```python
from build123d import *

# Parameters (mm, degrees)
SKETCH1_W           = 10
SKETCH1_H           = 10
BOSS_EXTRUDE1_DEPTH = 15
CUT_EXTRUDE1_DEPTH  = 0.3


with BuildPart() as part:
    # Sketch1 → Boss-Extrude1 (new body)
    with BuildSketch(Plane(origin=(0, 0, 0), x_dir=(1, 0, 0), z_dir=(0, 1, 0))):
        Rectangle(SKETCH1_W, SKETCH1_H)
        with BuildLine():
            Line((-1.658312395, 2.5), (1.658312395, 2.5))
            ThreePointArc((1.658312395, 2.5), (0, -3.043965134), (-1.658312395, 2.5))
        make_face(mode=Mode.SUBTRACT)
    extrude(amount=BOSS_EXTRUDE1_DEPTH)

    # Sketch2 → Cut-Extrude1 (cut)
    with BuildSketch(Plane.XY.offset(5)):
        with BuildLine():
            Line((-1.296362428, 9.754838654), (-0.6134698, 9.754838654))
            add(Edge.make_bspline(
                [(-0.6134698, 9.754838654), (-0.580041322, 9.754662904), (-0.515248611, 9.754322256), (-0.42102917, 9.749039125), (-0.332780359, 9.741835455), (-0.250476587, 9.730405362), (-0.174155884, 9.716613585), (-0.103588247, 9.699911769), (-0.038998075, 9.679885155), (0.038114662, 9.648038874), (0.126035323, 9.600715706), (0.221233715, 9.530787141), (0.302637955, 9.445254678), (0.372824272, 9.348772022), (0.428625391, 9.24263625), (0.468994689, 9.129377062), (0.494552564, 9.01045532), (0.497180998, 8.928812142), (0.498509367, 8.887550994)],
                knots=[0, 0, 0, 0, 0.00010027, 0.000194349, 0.000283026, 0.000365821, 0.000443519, 0.000515622, 0.000583254, 0.00064614, 0.000765662, 0.000881909, 0.000998927, 0.001118415, 0.001238844, 0.00135727, 0.001478274, 0.001601912, 0.001601912, 0.001601912, 0.001601912], degree=3))
            add(Edge.make_bspline(
                [(0.498509367, 8.887550994), (0.497416148, 8.848898438), (0.495267871, 8.772942521), (0.474725112, 8.661848412), (0.442564443, 8.556097193), (0.397859194, 8.456074808), (0.339757198, 8.364041195), (0.270898879, 8.279253929), (0.187822077, 8.205302872), (0.125578837, 8.163959969), (0.093962091, 8.142959648)],
                knots=[0, 0, 0, 0, 0.000115857, 0.00022767, 0.000337672, 0.000446877, 0.000555233, 0.000663318, 0.000773539, 0.000887324, 0.000887324, 0.000887324, 0.000887324], degree=3))
            add(Edge.make_bspline(
                [(0.093962091, 8.142959648), (0.133722519, 8.127694649), (0.209794066, 8.098488925), (0.314480078, 8.046853461), (0.404674923, 7.99069135), (0.481072069, 7.9293595), (0.546409724, 7.863250689), (0.603462666, 7.791395575), (0.65214404, 7.712856817), (0.693856964, 7.628453282), (0.72640572, 7.539046813), (0.750781624, 7.445476037), (0.764749073, 7.348076482), (0.766736714, 7.281791103), (0.767740136, 7.248328238)],
                knots=[0, 0, 0, 0, 0.000127722, 0.000244363, 0.000349599, 0.000445847, 0.000537565, 0.000627901, 0.000720503, 0.000814257, 0.000909859, 0.001005428, 0.001103887, 0.001204268, 0.001204268, 0.001204268, 0.001204268], degree=3))
            add(Edge.make_bspline(
                [(0.767740136, 7.248328238), (0.76676329, 7.214161366), (0.764841318, 7.146937088), (0.750661346, 7.048181953), (0.726652239, 6.953807006), (0.693581093, 6.863201824), (0.650418778, 6.776541689), (0.597890814, 6.693728425), (0.53525925, 6.615594095), (0.465196381, 6.541270471), (0.385934236, 6.474442684), (0.300418481, 6.414926977), (0.207572161, 6.365980915), (0.108920167, 6.324864894), (0.003355851, 6.293457695), (-0.108646757, 6.271485121), (-0.226991058, 6.256680084), (-0.308200809, 6.25546288), (-0.349848005, 6.254838654)],
                knots=[0, 0, 0, 0, 0.000102481, 0.000201635, 0.000298562, 0.000394165, 0.000490425, 0.000588455, 0.000687769, 0.000790423, 0.000894381, 0.000998232, 0.001102369, 0.001208616, 0.001318415, 0.001432129, 0.001550749, 0.00167562, 0.00167562, 0.00167562, 0.00167562], degree=3))
            Line((-0.349848005, 6.254838654), (-1.296362428, 6.254838654))
            Line((-1.296362428, 6.254838654), (-1.296362428, 9.754838654))
        make_face()
        with BuildLine():
            Line((-0.982259864, 9.395864295), (-0.982259864, 8.274069424))
            Line((-0.982259864, 8.274069424), (-0.771222204, 8.274069424))
            add(Edge.make_bspline(
                [(-0.771222204, 8.274069424), (-0.740373408, 8.274469347), (-0.680767249, 8.275242079), (-0.594447353, 8.277455596), (-0.514322334, 8.28365364), (-0.440530501, 8.289849902), (-0.373188057, 8.29992449), (-0.312444196, 8.311916612), (-0.257345599, 8.324599518), (-0.193806053, 8.346169004), (-0.121733105, 8.37804668), (-0.044900001, 8.427518516), (0.022834469, 8.486442869), (0.080031656, 8.554433831), (0.126843127, 8.629300017), (0.159356842, 8.709846897), (0.181404126, 8.794067029), (0.183395658, 8.851885282), (0.184406803, 8.881240898)],
                knots=[0, 0, 0, 0, 9.2559e-05, 0.000178842, 0.000258967, 0.000333616, 0.000400942, 0.000463093, 0.000519379, 0.000570374, 0.000664201, 0.000755025, 0.000843472, 0.000932526, 0.001020669, 0.001107124, 0.001192318, 0.001280185, 0.001280185, 0.001280185, 0.001280185], degree=3))
            add(Edge.make_bspline(
                [(0.184406803, 8.881240898), (0.183880622, 8.90066667), (0.182848462, 8.938772442), (0.17439516, 8.994321796), (0.160027585, 9.046565548), (0.141573292, 9.096219659), (0.115784603, 9.141731509), (0.08542114, 9.184674705), (0.04873545, 9.223586823), (0.006978137, 9.259956321), (-0.041030486, 9.292200849), (-0.095261777, 9.320441612), (-0.156449455, 9.343182389), (-0.223562309, 9.363098541), (-0.297633397, 9.377086835), (-0.37780795, 9.388740223), (-0.464742669, 9.394672965), (-0.524887772, 9.395458328), (-0.555977813, 9.395864295)],
                knots=[0, 0, 0, 0, 5.8261e-05, 0.000114285, 0.000168029, 0.000220632, 0.000272728, 0.000324483, 0.000378062, 0.000432741, 0.000490301, 0.000551137, 0.000615721, 0.000685833, 0.000760908, 0.00084162, 0.000928788, 0.00102206, 0.00102206, 0.00102206, 0.00102206], degree=3))
            Line((-0.555977813, 9.395864295), (-0.982259864, 9.395864295))
        make_face(mode=Mode.SUBTRACT)
        with BuildLine():
            Line((-0.982259864, 7.915095065), (-0.982259864, 6.613813013))
            Line((-0.982259864, 6.613813013), (-0.534944159, 6.613813013))
            add(Edge.make_bspline(
                [(-0.534944159, 6.613813013), (-0.502925233, 6.614196761), (-0.441212974, 6.614936383), (-0.352111744, 6.617350938), (-0.269528641, 6.622843214), (-0.193840505, 6.631489063), (-0.124230052, 6.640867512), (-0.061532349, 6.653478793), (-0.005239156, 6.667927754), (0.060035152, 6.690261926), (0.13353866, 6.724958397), (0.212749517, 6.777272623), (0.283175735, 6.839595931), (0.342980994, 6.911726845), (0.391993983, 6.990158172), (0.427649438, 7.073303522), (0.449640294, 7.15978905), (0.452302464, 7.218755762), (0.453637572, 7.248328238)],
                knots=[0, 0, 0, 0, 9.6064e-05, 0.000185151, 0.000267373, 0.000344257, 0.000413665, 0.000478015, 0.000536005, 0.000587888, 0.000684801, 0.000778918, 0.000871787, 0.000965866, 0.001059062, 0.00114827, 0.001236355, 0.001324974, 0.001324974, 0.001324974, 0.001324974], degree=3))
            add(Edge.make_bspline(
                [(0.453637572, 7.248328238), (0.453361467, 7.266821578), (0.452813712, 7.30350996), (0.444553097, 7.357425779), (0.432539228, 7.409651653), (0.417007794, 7.460329393), (0.394388327, 7.508542769), (0.367981782, 7.555245329), (0.33702038, 7.600498808), (0.288776214, 7.657711062), (0.21860423, 7.723628075), (0.118897454, 7.788165577), (0.005525156, 7.840213384), (-0.076702337, 7.86231286), (-0.119178935, 7.873728879)],
                knots=[0, 0, 0, 0, 5.5429e-05, 0.000109963, 0.000163198, 0.000216191, 0.000268588, 0.000322593, 0.000377046, 0.000432793, 0.000546889, 0.000664343, 0.000787646, 0.000919405, 0.000919405, 0.000919405, 0.000919405], degree=3))
            add(Edge.make_bspline(
                [(-0.119178935, 7.873728879), (-0.13620803, 7.877183963), (-0.173130623, 7.884675297), (-0.233338203, 7.892583001), (-0.302074072, 7.899628061), (-0.379496949, 7.904839218), (-0.46570479, 7.910225762), (-0.560881709, 7.912320583), (-0.664639024, 7.914819843), (-0.736631396, 7.915000977), (-0.774026691, 7.915095065)],
                knots=[0, 0, 0, 0, 5.2115e-05, 0.000112995, 0.000182062, 0.000259389, 0.000345767, 0.00044116, 0.000544948, 0.000657129, 0.000657129, 0.000657129, 0.000657129], degree=3))
            Line((-0.774026691, 7.915095065), (-0.982259864, 7.915095065))
        make_face(mode=Mode.SUBTRACT)
    extrude(amount=-CUT_EXTRUDE1_DEPTH, mode=Mode.SUBTRACT)


solid = part.part
```
Build history of the part. All positions in model axes, mm. A direction names the side the tool comes from. Coordinates: 2 decimals unless noted, no trailing zeros. Order: outer loops, then holes, each group sorted by start corner. A loop starts at its lowest first (then second) coordinate and runs counter-clockwise, first axis right, second up.
Item 1: Saw through at B-B on z = 0.75. List the corners of the cut face in (x, y), then the cut area to 3 significant figures.
Filled in:
outline: (-5, 0) - (-2.93, 0) - (-2.93, 15) - (-5, 15) - close; (2.93, 0) - (5, 0) - (5, 15) - (2.93, 15) - close
area: 62.1 mm2
Item 2: Saw through at A-A on y = 11.5. List the corners of the cut face in (x, z).
Filled in:
outline: (-5, -5) - (5, -5) - (5, 5) - (-5, 5) - close; hole (-1.66, -2.5) - (1.66, -2.5) arc R3.02 ccw (long way) to start
Item 3: Mould opens along Z. For faces 1 (the flat face through (0, 7, -2.5)), 2 (the flat face through (2.2, 0, -2.3)), 3 (the flat face through (0, 7, -5)), 4 (the flat face through (0, 7, 5)) say: released by +Z, released by -Z, zero draft, split by the parting line, or undercut.
Filled in:
face 1: undercut
face 2: zero draft
face 3: released by -Z
face 4: released by +Z
Item 4: Drop a flat-ended pin along its axis: pin 1 Ø1.5 at (x, z) = (-0.5, 0) entering from -Y. Give the stop position or say it passes through.
Filled in:
pin 1: passes through
Item 5: Drill centre lines: L1, parallel to Z at x = 0, y = 6; L2, parallel to Z at x = 0, y = 6.5; L3, parallel to X at y = 8.75, z = 0.75. Where is each one in solid material? Low to high.
Filled in:
L1: z = -5 to -2.5, 3.04 to 5
L2: z = -5 to -2.5, 3.04 to 4.7
L3: x = -5 to -2.93, 2.93 to 5
Item 6: Tool access for faces 5 (the flat face through (0, 8, 4.7)), 6 (the cylindrical face through (0.11, 7.4, 3.04)): list every direction of +Z, -Z, +X, -X, +Y, -Y with a clear straight run to the whole face (end or side of a thin tool).
Filled in:
face 5: +Z
face 6: +Y, -Y
